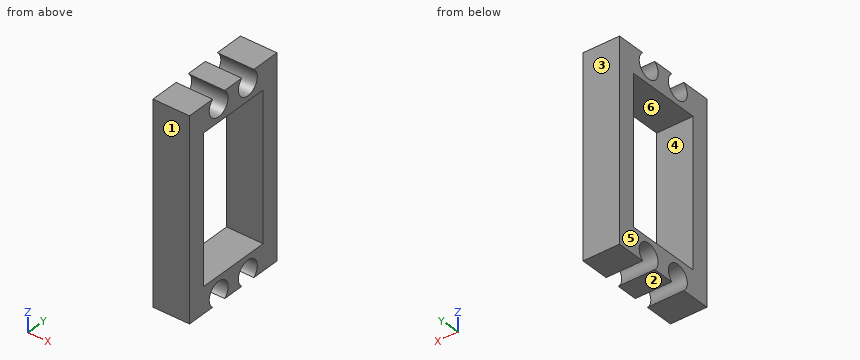
```python
from build123d import *

# Parameters (mm, degrees)
SKETCH1_W           = 54.5
SKETCH1_H           = 30
SKETCH1_W_2         = 40.25
SKETCH1_H_2         = 20.5
BOSS_EXTRUDE1_DEPTH = 10
CUT_EXTRUDE1_DEPTH  = 20


with BuildPart() as part:
    # Sketch1 → Boss-Extrude1 (new body)
    with BuildSketch(Plane(origin=(0, 0, 0), x_dir=(0, 0, -1), z_dir=(1, 0, 0))):
        with Locations((0, 10.75)):
            Rectangle(SKETCH1_W, SKETCH1_H)
        with Locations((0, 10.75)):
            Rectangle(SKETCH1_W_2, SKETCH1_H_2, mode=Mode.SUBTRACT)
    extrude(amount=BOSS_EXTRUDE1_DEPTH)

    # Sketch3 → Cut-Extrude1 (cut)
    with BuildSketch(Plane(origin=(10, 0, 0), x_dir=(0, 0, -1), z_dir=(1, 0, 0))):
        with BuildLine():
            Line((-27.25, 17.826655966), (-27.25, 13.673344034))
            ThreePointArc((-27.25, 13.673344034), (-21.5, 15.75), (-27.25, 17.826655966))
        make_face()
        with BuildLine():
            Line((27.25, 17.826655966), (27.25, 13.673344034))
            ThreePointArc((27.25, 13.673344034), (21.5, 15.75), (27.25, 17.826655966))
        make_face()
        with BuildLine():
            Line((27.25, 3.673344034), (27.25, 7.826655966))
            ThreePointArc((27.25, 7.826655966), (21.5, 5.75), (27.25, 3.673344034))
        make_face()
        with BuildLine():
            Line((-27.25, 3.673344034), (-27.25, 7.826655966))
            ThreePointArc((-27.25, 7.826655966), (-21.5, 5.75), (-27.25, 3.673344034))
        make_face()
    extrude(amount=-CUT_EXTRUDE1_DEPTH, mode=Mode.SUBTRACT)


solid = part.part
```
The listing builds one solid part. Answer for the finished solid, in the listing's coordinates (mm). Face numbers are marked on the shaded views. A direction names the side the tool comes from. Give positions to 0.01 mm unless a question says otherwise; leave off trailing zeros. Order: outer loops, then holes, each group sorted by start corner. A loop starts at its lowest first (then second) coordinate and runs counter-clockwise, first axis right, second up. Notation, with made-up numbers: M 16.25,-33.5 L 25.25,-33.5 A16 ccw 25.25,-14.5 Z; hole C 81.25,22 d8. An arc over 180 degrees is marked long. Put each result on its own line as item: value. Start each with the question number.
Item 1: The part is cut by section B-B, the plane z = -1. Determine the outline of the cut face in (x, y).
Item 2: The part is cut by section D-D, the plane z = -24.75. Determine the outline of the cut face in (x, y).
Item 3: The part is cut by section A-A, the plane y = 15.75. Determine the outline of the cut face in (x, z) (3 decimals).
Item 4: The part is cut by section C-C, the plane x = 8.75. Determine the outline of the cut face in (y, z) (3 decimals).
Item 5: Which of the six approach directions +Z, -Z, +X, -X, +Y, -Y give full straight-line access (tool end or side, diameter ignored) to the marked faces 5 and 6?
Item 6: Find the intervals of material crossed by line 1 along Y through (x, z) = (4.5, 24.75); line 2 along Z through (x, y) = (3.5, 19.75) (3 decimals); line 3 along Z through (x, y) = (6, 16) (3 decimals), in increasing order.
Item 7: For a pull along Y with two mould halves and no side action, classify the marked faces 1, 2, 3 and 4 as +Y half, -Y half, draft (parallel to the pull), parting line (faces both ways), or undercut.
Answer key:
1. outline: M 0,-4.25 L 10,-4.25 L 10,0.5 L 0,0.5 Z; M 0,21 L 10,21 L 10,25.75 L 0,25.75 Z
2. outline: M 0,-4.25 L 10,-4.25 L 10,2.5 L 0,2.5 Z; M 0,9 L 10,9 L 10,12.5 L 0,12.5 Z; M 0,19 L 10,19 L 10,25.75 L 0,25.75 Z
3. outline: M 0,-21.5 L 10,-21.5 L 10,-20.125 L 0,-20.125 Z; M 0,20.125 L 10,20.125 L 10,21.5 L 0,21.5 Z
4. outline: M -4.25,-27.25 L 3.673,-27.25 A3.25 cw long 7.827,-27.25 L 13.673,-27.25 A3.25 cw long 17.827,-27.25 L 25.75,-27.25 L 25.75,27.25 L 17.827,27.25 A3.25 cw long 13.673,27.25 L 7.827,27.25 A3.25 cw long 3.673,27.25 L -4.25,27.25 Z; hole M 0.5,-20.125 L 21,-20.125 L 21,20.125 L 0.5,20.125 Z
5. face 5: +Z, -Z, -X, +Y, -Y
5. face 6: +X, -X
6. line 1: y = -4.25 to 2.5, 9 to 12.5, 19 to 25.75
6. line 2: z = -27.25 to -20.125, 20.125 to 27.25
6. line 3: z = -21.51 to -20.125, 20.125 to 21.51
7. face 1: -Y half
7. face 2: draft
7. face 3: +Y half
7. face 4: undercut
